Verification items for the finished model (mm, model axes). A direction names the side the tool comes from. Round coordinates to 2 decimals unless told otherwise and drop trailing zeros. Write each loop counter-clockwise with the first axis right and the second up, starting at its lowest first coordinate (ties: lowest second). Pieces come first, ordered by that corner, then holes. Notation, with made-up numbers: M 49.5,-25.5 L 104.5,-25.5 A19 cw 104.5,4.5 Z; hole C 39.5,43.25 d6. An arc over 180 degrees is marked long. One line per question, with ' | ' between items. Start each with the question number.
Q1. Thickness scan on line 1 along Z through (x, y) = (-3.75, 4.5); line 2 along Y through (x, z) = (3, 11.25); line 3 along Z through (x, y) = (-3, -2.25). Record the ranges inside material, lowest first. Write a range as from..to.
Q2. Tool access check on faces 1 (the face through (-0.33, -6, 12.68)), 2 (the face through (0.156, 4.747, 5.381)), 3 (the face through (0, 1, 0)). Record the directions out of +Z, -Z, +X, -X, +Y, -Y that give a thin tool (end or side, any length) a straight path to the whole face; none if there is none.
Q3. Gauge pin test, flat ends, axial feed: pin 1 (2 mm diameter, centred on x = 4.5, z = 3, fed in from +Y); pin 2 (4 mm diameter, centred on y = 1.5, z = 8.5, fed in from -X); pin 3 (6 mm diameter, centred on x = -6, z = 11.5, fed in from +Y). Record the tip position at first contact, or that the pin passes through.
Q4. Cross-section at B-B (z = 10.2). Record the boundary of the cut face in (x, y).
Q5. Cross-section at C-C (y = -4). Record the boundary of the cut face in (x, z), then the cut area to 3 significant figures.
Q6. Cross-section at D-D (z = 4). Record the boundary of the cut face in (x, y).
Q7. Cross-section at A-A (x = 0). Record the boundary of the cut face in (y, z).
from build123d import *

# Parameters (mm, degrees)
F0_R          = 7.5
F1_DEPTH      = 2.3
F2_R          = 4.75
F3_DEPTH      = 11
F4_R          = 4.75
F6_START      = 3.3
F5_W          = 25.7861725986
F5_H          = 21.5545939282
F6_DEPTH      = 4.201
F7_R          = 2.5
F8_DEPTH      = 7
F8_DEPTH_BACK = 2
F9_R          = 0.5
F10_R         = 0.5


with BuildPart() as f1:
    # F0 (on Top) → F1 (new body)
    with BuildSketch(Plane.XY):
        Circle(F0_R)
    extrude(amount=F1_DEPTH)

    # F2 (on face) → F3 (join)
    with BuildSketch(Plane.XY.offset(2.3)):
        Circle(F2_R)
    extrude(amount=F3_DEPTH)

    # F4
    f4_edges = [f1.edges().sort_by_distance(p)[0] for p in [
        (-4.75, 0, 13.3),
    ]]
    fillet(f4_edges, radius=F4_R)

    # F5 (on Front) → F6 (cut)
    with BuildSketch(Plane.XZ.offset(F6_START)):
        with Locations((0.3588497639, 6.3574551605)):
            Rectangle(F5_W, F5_H)
    extrude(amount=F6_DEPTH, mode=Mode.SUBTRACT)

    # F7 (on face) → F8 (join, two sides)
    with BuildSketch(Plane.XZ.offset(3.3)) as f8_sk:
        with Locations((0, 10.2)):
            Circle(F7_R)
    extrude(amount=F8_DEPTH)
    extrude(f8_sk.sketch, amount=-F8_DEPTH_BACK)

    # F9
    f9_edges = [f1.edges().sort_by_distance(p)[0] for p in [
        (0, 7.5, 2.3),
    ]]
    fillet(f9_edges, radius=F9_R)

    # F10
    f10_edges = [f1.edges().sort_by_distance(p)[0] for p in [
        (-2.5, -10.3, 10.2),
    ]]
    fillet(f10_edges, radius=F10_R)


solid = f1.part
Determined:
1) line 1: z = 0..2.3 | line 2: y = -2.5..2.5 | line 3: z = 0..11.47
2) face 1: -Y | face 2: +Z | face 3: -Z, +X, -X, +Y, -Y
3) pin 1: stops at y = 6.19 | pin 2: stops at x = -4.75 | pin 3: stops at y = 3
4) outline: M -2.99,-3.3 L -2.5,-3.3 L -2.5,-9.8 A0.5 ccw -2,-10.3 L 2,-10.3 A0.5 ccw 2.5,-9.8 L 2.5,-3.3 L 2.99,-3.3 A4.45 ccw long Z
5) outline: C 0,10.2 d5 | area: 19.6 mm²
6) outline: M -3.42,-3.3 L 3.42,-3.3 A4.75 ccw long Z
7) outline: M -10.3,8.2 A0.5 ccw -9.8,7.7 L -3.3,7.7 L -3.3,0 L 7.5,0 L 7.5,1.8 A0.5 ccw 7,2.3 L 4.75,2.3 L 4.75,8.55 A4.75 ccw -2.31,12.7 L -9.8,12.7 A0.5 ccw -10.3,12.2 Z
